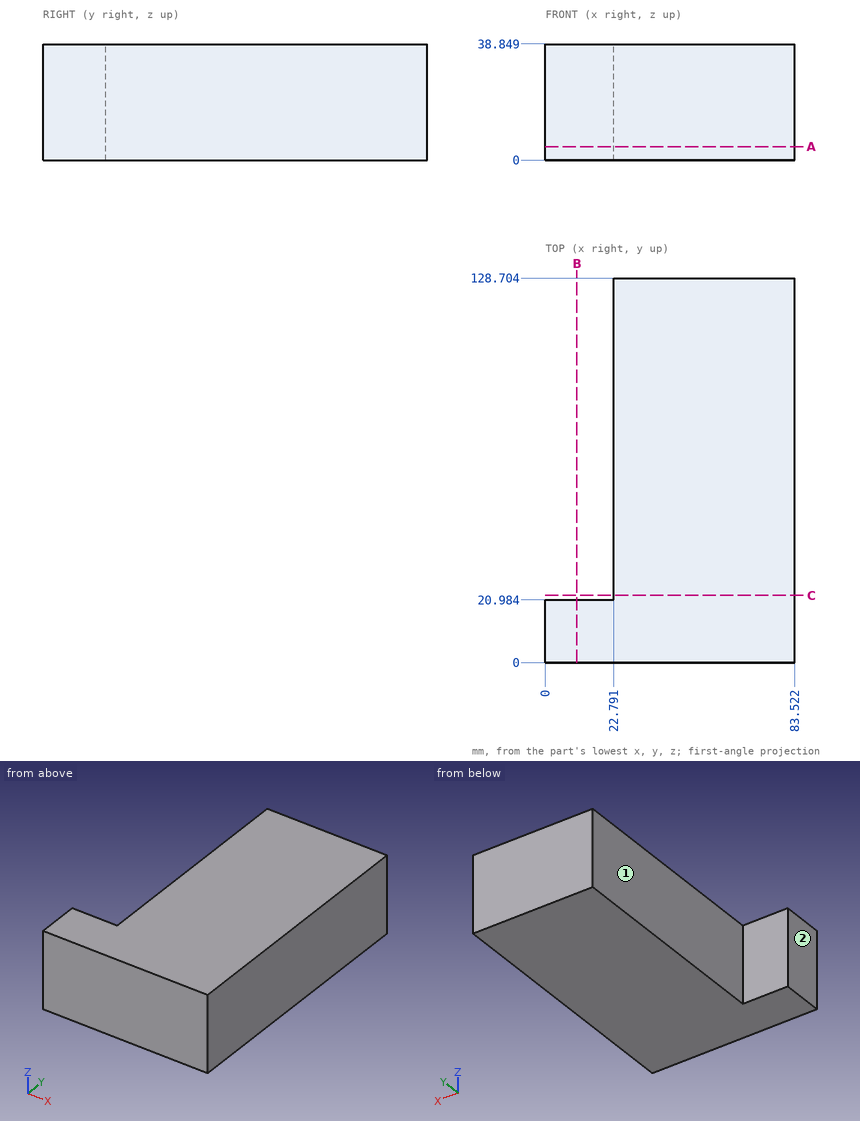
Design review of the part shown in the three views and the two pictorial views. Dimensions are in mm from the part's minimum x, y and z. A direction names the side the tool comes from. Give positions to 0.01 mm unless a question says otherwise; leave off trailing zeros. Loops run counter-clockwise (first coordinate to the right, second up) from the corner with the lowest first, then second, coordinate; pieces in that order, holes last. Notation, with made-up numbers: (-32, -7.75) -> (4, -7.75) arc R20 ccw to (4, 27.25) -> close; hole circle Ø7 at (54.25, 73). An arc over 180 degrees is marked (long way). One line per question, with ' | ' between items.
1) We need section B-B (x = 10.5). Write out the cut boundary in (y, z).
Resolved:
outline: (0, 0) -> (20.98, 0) -> (20.98, 38.85) -> (0, 38.85) -> close
2) We need section C-C (y = 22.5). Write out the cut boundary in (x, z), plus the area to 3 significant figures.
Resolved:
outline: (22.79, 0) -> (83.52, 0) -> (83.52, 38.85) -> (22.79, 38.85) -> close | area: 2,360 mm2
3) To check wall thickness, follow probe 1 along X at (y, z) = (98, 20.5); probe 2 along Y at (x, z) = (13, 2.5). State the ranges of each line that lie inside material, in increasing order.
Resolved:
probe 1: x = 22.79 to 83.52 | probe 2: y = 0 to 20.98
4) We need section A-A (z = 4.5). Write out the cut boundary in (x, y), plus the area to 3 significant figures.
Resolved:
outline: (0, 0) -> (83.52, 0) -> (83.52, 128.7) -> (22.79, 128.7) -> (22.79, 20.98) -> (0, 20.98) -> close | area: 8,290 mm2
5) For the marked faces 1 and 2, list the 3-axis set-ups (+Z, -Z, +X, -X, +Y, -Y) from which the entire face can be reached by the end or side of a thin tool; tool diameter is ignored.
Resolved:
face 1: +Z, -Z, -X, +Y | face 2: +Z, -Z, -X, +Y, -Y
6) Insertion check: pin 1 Ø19.5 at (y, z) = (99.5, 18.5) entering from -X. The pin has a flat end and moves straight along its axis. Give the tip position at first contact, or say it passes through.
Resolved:
pin 1: stops at x = 22.79
